Build history of the part. All positions in model axes, mm. Face numbers are marked on the shaded views. A direction names the side the tool comes from. Round coordinates to 2 decimals unless told otherwise and drop trailing zeros. Loops run counter-clockwise (first coordinate to the right, second up) from the corner with the lowest first, then second, coordinate; pieces in that order, holes last. Notation, with made-up numbers: M -24,11.5 L -4,11.5 A14 cw -4,21.5 Z; hole C -36.5,75 d8. An arc over 180 degrees is marked long. Use one line per item in the form item = value. Start each with the question number.
```python
from build123d import *

# Parameters (mm, degrees)
F0_W     = 76.2
F0_H     = 63.5
F1_DEPTH = 25.4
F3_DEPTH = 50.8
F4_W     = 63.5
F4_H     = 25.4
F5_DEPTH = 63.5


with BuildPart() as f1:
    # F0 (on Top) → F1 (new body)
    with BuildSketch(Plane.XY):
        with Locations((0.813381, -8.013141)):
            Rectangle(F0_W, F0_H)
    extrude(amount=F1_DEPTH)

    # F2 (on face) → F3 (join)
    with BuildSketch(Plane.XY.offset(25.4)):
        Polygon((-37.286619, 23.736859), (-37.286619, -39.763141), (-11.886619, -39.763141), (-11.886619, -1.663141), (26.213381, -1.663141), (26.213381, 23.736859), align=None)
    extrude(amount=F3_DEPTH)

    # F4 (on face) → F5 (join)
    with BuildSketch(Plane(origin=(-37.286619, 0, 0), x_dir=(0, -1, 0), z_dir=(-1, 0, 0))):
        with Locations((8.013141, 63.5)):
            Rectangle(F4_W, F4_H)
    extrude(amount=F5_DEPTH)


solid = f1.part
```
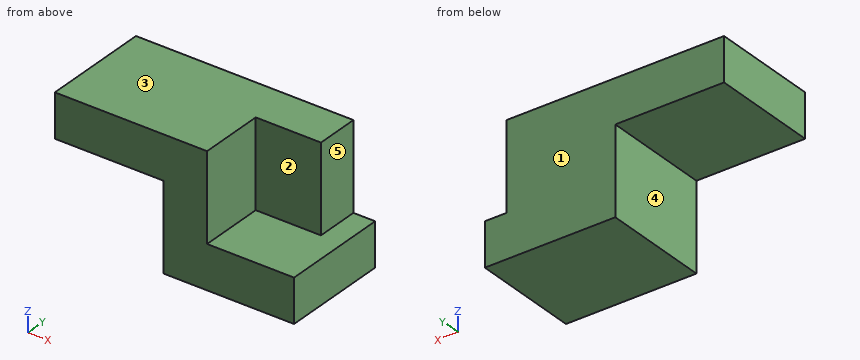
Q1. Drop flat-ended pins along their axis: P1, Ø19, axis at x = -78, y = -22.5, coming from the -Z side; P2, Ø5, axis at x = -5.5, z = 46, coming from the -Y side; P3, Ø20.5, axis at y = 7, z = 54, coming from the +X side; P4, Ø6, axis at x = -6, y = -19, coming from the -Z side. Give the stop position or say it passes through.
Q2. Wall check: probe 1 along X at (y, z) = (5, 8.5); probe 2 along X at (y, z) = (-37, 34); probe 3 along Z at (x, y) = (-81, -31). Give the ranges that are in metal, low to high.
Q3. Saw through at B-B (z = 60.5). Give the cut face in (x, y).
Q4. Tool access for the marked faces 1, 2, 3, 4 and 5: list every direction of +Z, -Z, +X, -X, +Y, -Y with a clear straight run to the whole face (end or side of a thin tool).
Q5. Saw through at D-D (y = 16). Give the cut face in (x, z).
Q6. Saw through at C-C (x = -65). Give the cut face in (y, z).
Q7. Saw through at A-A (y = -23). Give the cut face in (x, z).
Filled in:
q1.P1 = 50.8
q1.P2 = -1.66
q1.P3 = 26.21
q1.P4 = 0
q2.probe_1 = -37.29 to 38.91
q2.probe_2 = -37.29 to -11.89
q2.probe_3 = 50.8 to 76.2
q3.outline = M -100.79,-39.76 L -11.89,-39.76 L -11.89,-1.66 L 26.21,-1.66 L 26.21,23.74 L -100.79,23.74 Z
q4.face_1 = +Z, -Z, +X, -X, +Y
q4.face_2 = +Z, +X, -Y
q4.face_3 = +Z, +X, -X, +Y, -Y
q4.face_4 = -Z, -X, +Y, -Y
q4.face_5 = +Z, +X, +Y, -Y
q5.outline = M -100.79,50.8 L -37.29,50.8 L -37.29,0 L 38.91,0 L 38.91,25.4 L 26.21,25.4 L 26.21,76.2 L -100.79,76.2 Z
q6.outline = M -39.76,50.8 L 23.74,50.8 L 23.74,76.2 L -39.76,76.2 Z
q7.outline = M -100.79,50.8 L -37.29,50.8 L -37.29,0 L 38.91,0 L 38.91,25.4 L -11.89,25.4 L -11.89,76.2 L -100.79,76.2 Z
